The model under review builds one solid part; all positions refer to its coordinate system, in mm. A direction names the side the tool comes from. Round coordinates to 2 decimals unless told otherwise and drop trailing zeros. Order: outer loops, then holes, each group sorted by start corner. A loop starts at its lowest first (then second) coordinate and runs counter-clockwise, first axis right, second up. Notation, with made-up numbers: (11, -22.75) -> (59, -22.75) arc R33 cw to (59, 13.25) -> close; hole circle Ø5 at (-34.75, 22). An arc over 180 degrees is marked (long way). Put each result on its own line as item: value. Start each with the question number.
Autodesk Inventor part; units mm, degrees
ref_plane "YZ Plane" through (0, 0, 0) normal (1, 0, 0) x (0, 1, 0)
ref_plane "XY Plane" through (0, 0, 0) normal (0, 0, 1) x (1, 0, 0)
sketch "Sketch1" plane through (0, 0, 0) normal (1, 0, 0) x (0, 1, 0)
  circle A0 centre (0, 0) radius 16.5
  circle A1 centre (0, 0) radius 19.5
  dimension "d0" = 33
  dimension "d1" = 3
extrude "Extrusion1" add sketch "Sketch1" along normal blind 20.75 contours A0 | A1
sketch "Sketch2" plane through (0, 0, 0) normal (-1, 0, 0) x (0, 0, 1)
  circle A0 centre (0, 0) radius 19.5
  circle A1 centre (0, 0) radius 16.5
  dimension "d4" = 33
extrude "Extrusion2" cut sketch "Sketch2" against normal blind 25 contours A1
ref_plane "Work Plane2" through (0, -19.5, 0) normal (0, 1, 0) x (-1, 0, 0)
sketch "Sketch6" plane through (20.75, 0, 0) normal (1, 0, 0) x (0, 0, -1)
  circle A0 centre (0, 0) radius 10.25
  circle A1 centre (0, 0) radius 19.5
  circle A2 centre (0, 0) radius 13
  dimension "d14" = 26
extrude "Extrusion5" add sketch "Sketch6" against normal blind 30 contours A2
sketch "Sketch7" plane through (20.75, 0, 0) normal (1, 0, 0) x (0, 0, -1)
  circle A0 centre (0, 0) radius 19.5
  circle A1 centre (0, 0) radius 19.5
  circle A2 centre (0, 0) radius 16.5
  circle A3 centre (0, 0) radius 10.25
  dimension "d23" = 20.5
extrude "Extrusion7" add sketch "Sketch7" against normal blind 2 contours A2
properties part number "union pvc tubo"
Q1. Draft analysis for pull direction Z (two halves, no side actions). For faces 3 (the face through (10.23, -2.539, -19.334)), 4 (the face through (-9.25, 4, -10)), 5 (the face through (18.75, -13.4, 0.1)), state which applies: +Z half, -Z half, draft (parallel to the pull), parting line (faces both ways), or undercut.
Q2. Clearance check with flat-ended pins moving along their axes: pin 1 Ø18.5 at (y, z) = (0, 0) entering from +X; pin 2 Ø4 at (x, y) = (-3.5, 12) entering from +Z; pin 3 Ø8 at (x, z) = (-6, 2.5) entering from +Y; pin 4 Ø10 at (x, z) = (15, 12) entering from -Y. State where each tip first meets the part, or that it passes through.
Q3. Take a section at C-C on x = 14.25. Give the boundary of the cut face in (y, z).
Q4. Take a section at D-D on x = -3.5. Give the boundary of the cut face in (y, z).
Q5. Take a section at A-A on y = 0. Give the boundary of the cut face in (x, z).
Q6. For faces 1 (the face through (9.24, -6.32, 15.24)), 2 (the face through (5.96, -10.006, 2.222)), list the 3-axis set-ups (+Z, -Z, +X, -X, +Y, -Y) from which the entire face can be reached by the end or side of a thin tool; tool diameter is ignored.
Q7. Wall thickness on probe 1 along Y at (x, z) = (4, 8); probe 2 along Y at (x, z) = (9.75, 11.5); probe 3 along Z at (x, y) = (7.25, 3.5): over which ranges is each line inside the solid? List them lowest first. Write a range as [from, to].
Calculated:
1. face 3: parting line
1. face 4: draft
1. face 5: undercut
2. pin 1: passes through
2. pin 2: stops at z = 8.31
2. pin 3: stops at y = 13
2. pin 4: stops at y = -18.2
3. outline: circle Ø39 at (0, 0); circle Ø26 at (0, 0); hole circle Ø33 at (0, 0); hole circle Ø20.5 at (0, 0)
4. outline: circle Ø26 at (0, 0); hole circle Ø20.5 at (0, 0)
5. outline: (-9.25, -13) -> (18.75, -13) -> (18.75, -16.5) -> (0, -16.5) -> (0, -19.5) -> (20.75, -19.5) -> (20.75, -10.25) -> (-9.25, -10.25) -> close; (-9.25, 10.25) -> (20.75, 10.25) -> (20.75, 19.5) -> (0, 19.5) -> (0, 16.5) -> (18.75, 16.5) -> (18.75, 13) -> (-9.25, 13) -> close
6. face 1: -X
6. face 2: +X, -X
7. probe 1: y = [-17.78, -14.43], [-10.25, -6.41], [6.41, 10.25], [14.43, 17.78]
7. probe 2: y = [-15.75, -11.83], [-6.06, 6.06], [11.83, 15.75]
7. probe 3: z = [-19.18, -16.12], [-12.52, -9.63], [9.63, 12.52], [16.12, 19.18]
